Autodesk Inventor part; units mm, degrees
ref_plane "YZ Plane" through (0, 0, 0) normal (1, 0, 0) x (0, 1, 0)
ref_plane "XZ Plane" through (0, 0, 0) normal (0, 1, 0) x (-1, 0, 0)
ref_plane "XY Plane" through (0, 0, 0) normal (0, 0, 1) x (1, 0, 0)
sketch "Sketch1" plane through (0, 0, 0) normal (1, 0, 0) x (0, 1, 0)
  line L0 (0, 0) -> (0, -44.3) construction
  line L1 (10.65, -10.65) -> (10.65, -33.65)
  line L2 (-10.65, -33.65) -> (-10.65, -10.65)
  arc A0 (10.65, -10.65) -> (-10.65, -10.65) centre (0, -10.65) ccw
  arc A1 (-10.65, -33.65) -> (10.65, -33.65) centre (0, -33.65) ccw
  point P0 (0, -22.15)
  dimension "d0" = 44.3
  dimension "d1" = 21.3
extrude "Extrusion1" add sketch "Sketch1" against normal blind 55
fillet "Fillet1" radius 4 4 edges at (0, 0, 0) (0, -10.65, -22.15) (0, 0, -44.3) (0, 10.65, -22.15)
properties part number "Among Us Goggles"
CAD build for the part. Positions are in the model's coordinates, mm. Round coordinates to 2 decimals unless told otherwise and drop trailing zeros. Write each loop counter-clockwise with the first axis right and the second up, starting at its lowest first coordinate (ties: lowest second). Pieces come first, ordered by that corner, then holes. Notation, with made-up numbers: (55.5, 40) - (106.5, 40) arc R23 cw to (106.5, 71) - close; hole circle Ø1 at (12, -21.75). An arc over 180 degrees is marked (long way). Return JSON: item names as keys, results as strings. Group by question number.
Item 1: Probe probe 1 along Z at (x, y) = (-47.5, -0.5); probe 2 along Y at (x, z) = (-14.5, -10.5); probe 3 along X at (y, z) = (-7, -20.5). List the from-to ranges inside material, lowest first.
Item 2: Flat gauge pins, fed straight in: pin 1 Ø5 at (x, y) = (-41, 8.5) entering from +Z; pin 2 Ø4 at (x, z) = (-32.5, -39) entering from -Y; pin 3 Ø1.5 at (x, y) = (-48.5, 3.5) entering from -Z. Where does each tip first touch, or does it go through?
Item 3: Band-saw the part on A-A on x = -41.5. List the corners of the cut face in (y, z), plus the area to 3 significant figures.
Resolved:
{
 "1": {"probe 1": "z = -44.29 to -0.01", "probe 2": "y = -10.65 to 10.65", "probe 3": "x = -55 to -0.02"},
 "2": {"pin 1": "stops at z = -1.85", "pin 2": "stops at y = -10.11", "pin 3": "stops at z = -43.94"},
 "3": {"outline": "(-10.65, -33.65) arc R10.65 ccw to (10.65, -33.65) - (10.65, -10.65) arc R10.65 ccw to (-10.65, -10.65) - close", "area": "846 mm²"}
}
